```python
from build123d import *

# Parameters (mm, degrees)
SKETCH1_W                = 50
SKETCH1_H                = 50
PLATE_BODY_DEPTH         = 2
SKETCH2_R                = 4.1
SHAFT_BEARINGS_DEPTH     = 3
SKETCH3_R                = 1
BEARING_BOLT_HOLES_DEPTH = 3
CUT_EXTRUDE1_DEPTH       = 3


with BuildPart() as part:
    # Sketch1 → plate_body (new body)
    with BuildSketch(Plane.XY):
        with Locations((25, 25)):
            Rectangle(SKETCH1_W, SKETCH1_H)
    extrude(amount=PLATE_BODY_DEPTH)

    # Sketch2 → shaft_bearings (cut, through all)
    with BuildSketch(Plane.XY.offset(2)):
        with Locations((6, 25)):
            Circle(SKETCH2_R)
        with Locations((44, 25)):
            Circle(SKETCH2_R)
    extrude(amount=-SHAFT_BEARINGS_DEPTH, mode=Mode.SUBTRACT)

    # Sketch3 → bearing_bolt_holes (cut, through all)
    with BuildSketch(Plane.XY.offset(2)):
        with Locations((6, 31)):
            Circle(SKETCH3_R)
        with Locations((6, 19)):
            Circle(SKETCH3_R)
        with Locations((44, 31)):
            Circle(SKETCH3_R)
        with Locations((44, 19)):
            Circle(SKETCH3_R)
    extrude(amount=-BEARING_BOLT_HOLES_DEPTH, mode=Mode.SUBTRACT)

    # Sketch4 → Cut-Extrude1 (cut, through all)
    with BuildSketch(Plane.XY.offset(2)):
        with BuildLine():
            Line((26.75, 42.5), (26.75, 7.5))
            ThreePointArc((26.75, 7.5), (25, 5.75), (23.25, 7.5))
            Line((23.25, 7.5), (23.25, 42.5))
            ThreePointArc((23.25, 42.5), (25, 44.25), (26.75, 42.5))
        make_face()
    extrude(amount=-CUT_EXTRUDE1_DEPTH, mode=Mode.SUBTRACT)


solid = part.part
```
Geometry check sheet. Reference: the model listing, model coordinates, mm. A direction names the side the tool comes from. Give positions to 0.01 mm unless a question says otherwise; leave off trailing zeros. Loops run counter-clockwise (first coordinate to the right, second up) from the corner with the lowest first, then second, coordinate; pieces in that order, holes last. Notation, with made-up numbers: M 14.25,26.25 L 24.25,26.25 A30 ccw 24.25,58.25 Z; hole C -37,37 d8. An arc over 180 degrees is marked long. Answer as CSV lines item,"result".
Item 1: Cross-section at C-C on z = 1.2. Record the cut outline in (x, y), and give its area (3 significant figures).
Values:
outline,"M 0,0 L 50,0 L 50,50 L 0,50 Z; hole C 6,25 d8.2; hole C 6,19 d2; hole C 6,31 d2; hole M 23.25,7.5 A1.75 ccw 26.75,7.5 L 26.75,42.5 A1.75 ccw 23.25,42.5 Z; hole C 44,25 d8.2; hole C 44,19 d2; hole C 44,31 d2"
area,"2,250 mm²"
Item 2: Release check for a two-part mould opening along X. For faces 3 (the flat face through (25, 0, 1)), 4 (the flat face through (50, 25, 1)), 5 (the cylindrical face through (24.96, 44.25, 1.01)), 6 (the flat face through (0, 25, 1)) record: pulls with the +X half, pulls with the -X half, needs draft (parallel to the pull), parting line crosses it, or undercut.
Values:
face 3,"needs draft"
face 4,"pulls with the +X half"
face 5,"undercut"
face 6,"pulls with the -X half"
Item 3: Cross-section at D-D on x = 44. Record the cut outline in (y, z).
Values:
outline,"M 0,0 L 18,0 L 18,2 L 0,2 Z; M 20,0 L 20.9,0 L 20.9,2 L 20,2 Z; M 29.1,0 L 30,0 L 30,2 L 29.1,2 Z; M 32,0 L 50,0 L 50,2 L 32,2 Z"
Item 4: Cross-section at B-B on y = 31. Record the cut outline in (x, z).
Values:
outline,"M 0,0 L 5,0 L 5,2 L 0,2 Z; M 7,0 L 23.25,0 L 23.25,2 L 7,2 Z; M 26.75,0 L 43,0 L 43,2 L 26.75,2 Z; M 45,0 L 50,0 L 50,2 L 45,2 Z"
Item 5: Cross-section at A-A on x = 25. Record the cut outline in (y, z).
Values:
outline,"M 0,0 L 5.75,0 L 5.75,2 L 0,2 Z; M 44.25,0 L 50,0 L 50,2 L 44.25,2 Z"
Item 6: Material ranges on line 1 (Y direction, x = 44, z = 1.4); line 2 (X direction, y = 28, z = 0.5); line 3 (X direction, y = 22.5, z = 1.8), recorded low to high.
Values:
line 1,"y = 0 to 18, 20 to 20.9, 29.1 to 30, 32 to 50"
line 2,"x = 0 to 3.21, 8.79 to 23.25, 26.75 to 41.21, 46.79 to 50"
line 3,"x = 0 to 2.75, 9.25 to 23.25, 26.75 to 40.75, 47.25 to 50"
Item 7: Access from +Z, -Z, +X, -X, +Y, -Y to the whole of each face (thin tool, end or side, straight path). Record for faces 1 (the flat face through (26.75, 25, 1)), 2 (the flat face through (19, 25, 0)).
Values:
face 1,"+Z, -Z"
face 2,"-Z, +X, -X, +Y, -Y"
